Could you check a few things on this model? Use its own coordinates, in mm. Give positions to 0.01 mm unless a question says otherwise; leave off trailing zeros. Order: outer loops, then holes, each group sorted by start corner. A loop starts at its lowest first (then second) coordinate and runs counter-clockwise, first axis right, second up. Notation, with made-up numbers: M 10.5,62.25 L 53.5,62.25 A8 cw 53.5,77.25 Z; hole C 15,52 d8. An arc over 180 degrees is marked long. Answer in a Markdown table with one row per item. Add a question column.
```python
from build123d import *

# Parameters (mm, degrees)
BOSS_EXTRUDE1_DEPTH = 300
CHAMFER1_SIZE       = 0.3
LPATTERN1_COUNT     = 7
LPATTERN1_PITCH     = 40


with BuildPart() as part:
    # Sketch1 → Boss-Extrude1 (new body)
    with BuildSketch(Plane.XY):
        with BuildLine():
            Line((0, 8), (12, 8))
            Line((12, 8), (12, 6.75))
            Line((12, 6.75), (12, 6.559016994))
            ThreePointArc((12, 6.559016994), (11.706107374, 6.475528258), (11.5, 6.25))
            Line((11.5, 6.25), (11, 6.25))
            Line((11, 6.25), (11, 5.75))
            Line((11, 5.75), (11.5, 5.75))
            ThreePointArc((11.5, 5.75), (11.706107374, 5.524471742), (12, 5.440983006))
            Line((12, 5.440983006), (12, 5.25))
            Line((12, 5.25), (12, 0))
            Line((12, 0), (0, 0))
            Line((0, 0), (0, 5.25))
            Line((0, 5.25), (0, 5.440983006))
            ThreePointArc((0, 5.440983006), (0.293892626, 5.524471742), (0.5, 5.75))
            Line((0.5, 5.75), (1, 5.75))
            Line((1, 5.75), (1, 6.25))
            Line((1, 6.25), (0.5, 6.25))
            ThreePointArc((0.5, 6.25), (0.293892626, 6.475528258), (0, 6.559016994))
            Line((0, 6.559016994), (0, 6.75))
            Line((0, 6.75), (0, 8))
        make_face()
    extrude(amount=BOSS_EXTRUDE1_DEPTH)

    # Chamfer1
    chamfer1_edges = [part.edges().sort_by_distance(p)[0] for p in [
        (12, 2.720491503, 300),
        (11.706107374, 5.524471742, 300),
        (0, 2.720491503, 0),
        (0.293892626, 5.524471742, 0),
        (0.75, 5.75, 0),
        (1, 6, 0),
        (0.75, 6.25, 0),
        (11.25, 5.75, 300),
        (0.293892626, 6.475528258, 0),
        (0, 7.279508497, 0),
        (6, 8, 0),
        (12, 7.279508497, 0),
        (11.706107374, 6.475528258, 0),
        (11, 6, 300),
        (11.25, 6.25, 0),
        (11, 6, 0),
        (11.25, 5.75, 0),
        (11.706107374, 5.524471742, 0),
        (12, 2.720491503, 0),
        (6, 0, 0),
        (11.25, 6.25, 300),
        (11.706107374, 6.475528258, 300),
        (12, 7.279508497, 300),
        (0, 8, 150),
        (12, 8, 150),
        (12, 0, 150),
        (0, 0, 150),
        (6, 8, 300),
        (0, 2.720491503, 300),
        (0, 7.279508497, 300),
        (0.293892626, 6.475528258, 300),
        (0.75, 6.25, 300),
        (1, 6, 300),
        (0.75, 5.75, 300),
        (0.293892626, 5.524471742, 300),
        (6, 0, 300),
    ]]
    chamfer(chamfer1_edges, length=CHAMFER1_SIZE)

    # Sketch3 → CBORE for M5 Hex Head Bolt1 (revolve, cut)
    with BuildSketch(Plane(origin=(6, 8, 15), x_dir=(0, 0, 1), z_dir=(1, 0, 0))):
        Polygon((0, 0), (0, 8), (2.5, 8), (2.25, 7.75), (2.25, 4.5), (4, 4.5), (4, 0.25), (4.25, 0), align=None)
    cbore_for_m5_hex_head_bolt1 = revolve(axis=Axis((6, 14.35, 15), (0, -1, 0)), mode=Mode.SUBTRACT)

    # LPattern1: CBORE for M5 Hex Head Bolt1 ×7
    with Locations(*[(0, 0, i * LPATTERN1_PITCH) for i in range(1, LPATTERN1_COUNT)]):
        add(cbore_for_m5_hex_head_bolt1, mode=Mode.SUBTRACT)


solid = part.part
```
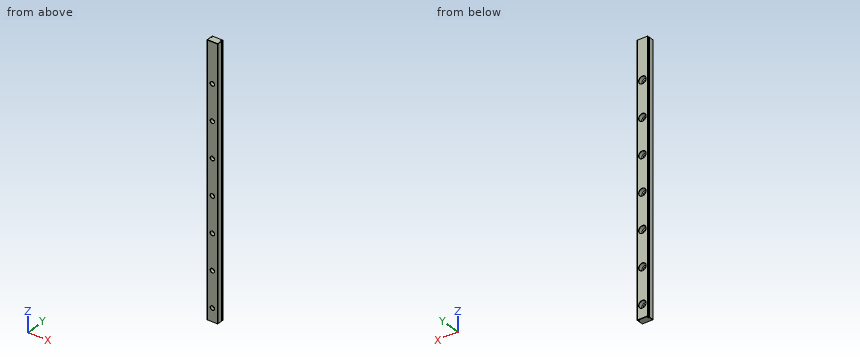
1. Suppose I cut it at C-C on z = 244.5. List the corners of the cut face in (x, y) for me, plus the area to 3 significant figures.
2. If I drill on line 1 along X through (y, z) = (2.2, 55); line 2 along X through (y, z) = (6.05, 215); line 3 along Y through (x, z) = (11.5, 255.5), over which ranges is the centre line in solid material (lowest first)? Write a range as [from, to].
3. Suppose I cut it at B-B on x = 6. Count the separate pieces of the cut face and the enclosed holes in it, plus the area to 3 significant figures.
4. Will these pins go through, and if not, where does the flat tip stop? P1, Ø4, axis at x = 6, z = 255, coming from the -Y side; P2, Ø7, axis at x = 6, z = 15, coming from the +Y side.
5. Suppose I cut it at A-A on y = 2. List the corners of the cut face in (x, z) for me, plus the area to 3 significant figures.
Findings below:
| question | item | result |
|---|---|---|
| 1 | outline | M 0,0.3 L 0.3,0 L 11.7,0 L 12,0.3 L 12,5.44 A0.56 cw 11.5,5.75 L 11,5.75 L 11,6.25 L 11.5,6.25 A0.56 cw 12,6.56 L 12,7.7 L 11.7,8 L 0.3,8 L 0,7.7 L 0,6.56 A0.56 cw 0.5,6.25 L 1,6.25 L 1,5.75 L 0.5,5.75 A0.56 cw 0,5.44 Z |
| 1 | area | 94.4 mm2 |
| 2 | line 1 | [0, 3.75], [8.25, 12] |
| 2 | line 2 | [1, 2], [10, 11] |
| 2 | line 3 | [0, 5.75], [6.25, 8] |
| 3 | separate pieces | 8 |
| 3 | enclosed holes | 0 |
| 3 | area | 2,040 mm2 |
| 4 | P1 | through |
| 4 | P2 | y = 3.5 |
| 5 | outline | M 0,0.3 L 0.3,0 L 11.7,0 L 12,0.3 L 12,299.7 L 11.7,300 L 0.3,300 L 0,299.7 Z; hole C 6,15 d4.5; hole C 6,55 d4.5; hole C 6,95 d4.5; hole C 6,135 d4.5; hole C 6,175 d4.5; hole C 6,215 d4.5; hole C 6,255 d4.5 |
| 5 | area | 3,490 mm2 |
